Autodesk Inventor part; units mm, degrees
ref_plane "YZ Plane" through (0, 0, 0) normal (1, 0, 0) x (0, 1, 0)
ref_plane "XZ Plane" through (0, 0, 0) normal (0, 1, 0) x (-1, 0, 0)
ref_plane "XY Plane" through (0, 0, 0) normal (0, 0, 1) x (1, 0, 0)
sketch "Esboço1" plane through (0, 0, 0) normal (0, 1, 0) x (-1, 0, 0)
  line L0 (20, 75) -> (-20, 75)
  line L1 (-20, 75) -> (-20, -75)
  line L2 (-20, -75) -> (20, -75)
  line L3 (20, -75) -> (20, 75)
  line L4 (7.1, 63.25) -> (7.1, 18.19) construction
  circle A0 centre (7.1, 16.44) radius 1.75 construction
  circle A1 centre (7.1, 65) radius 1.75 construction
  line L5 (7.1, 65) -> (7.1, 63.25) construction
  line L6 (7.1, 16.44) -> (7.1, 18.19) construction
  circle A2 centre (7.1, 16.44) radius 1.45
  circle A3 centre (7.1, 65) radius 1.45
  line L7 (14.5, 62.22) -> (-14.5, 62.22) construction
  line L8 (-14.5, 62.22) -> (-14.5, 19.22) construction
  line L9 (-14.5, 19.22) -> (14.5, 19.22) construction
  line L10 (14.5, 19.22) -> (14.5, 62.22) construction
  line L11 (11.1, 61) -> (3.1, 61) construction
  line L12 (3.1, 61) -> (3.1, 69) construction
  line L13 (3.1, 69) -> (11.1, 69) construction
  line L14 (11.1, 69) -> (11.1, 61) construction
  line L15 (11.1, 61) -> (3.1, 69) construction
  line L16 (3.1, 61) -> (11.1, 69) construction
  line L17 (3.1, 20.44) -> (11.1, 20.44) construction
  line L18 (11.1, 20.44) -> (11.1, 12.44) construction
  line L19 (11.1, 12.44) -> (3.1, 12.44) construction
  line L20 (3.1, 12.44) -> (3.1, 20.44) construction
  line L21 (3.1, 20.44) -> (11.1, 12.44) construction
  line L22 (11.1, 20.44) -> (3.1, 12.44) construction
  line L23 (7.1, 40.72) -> (7.6918, 40.72) construction
  line L24 (14.5, 40.72) -> (22.5062, 40.72) construction
  line L25 (7.1, -1.12) -> (7.1, -24.28) construction
  circle A4 centre (7.1, -1.12) radius 1.45
  circle A5 centre (7.1, -24.28) radius 1.45
  circle A6 centre (7.1, -41.84) radius 1.45
  circle A7 centre (7.1, -65) radius 1.45
  line L26 (7.1, -41.84) -> (7.1, -65) construction
  line L27 (7.1, 16.44) -> (7.1, -1.12) construction
  line L28 (7.1, -24.28) -> (7.1, -41.84) construction
  line L29 (0, 62.22) -> (0, 19.22) construction
  line L30 (0, 75) -> (0, 85.6082) construction
  point P0 (0, 0)
  dimension "d5" = 3.5
  dimension "d6" = 3.5
  dimension "d0" = 150
  dimension "d1" = 40
  dimension "d2" = 20
  dimension "d3" = 75
  dimension "d4" = 45.06
  dimension "d7" = 2.9
  dimension "d8" = 2.9
  dimension "d9" = 48.56
  dimension "d10" = 29
  dimension "d11" = 8
  dimension "d12" = 8
  dimension "d13" = 8
  dimension "d14" = 8
  dimension "d15" = 3.4
  dimension "d16" = 43
  dimension "d17" = 2.9
  dimension "d18" = 2.9
  dimension "d19" = 23.16
  dimension "d20" = 2.9
  dimension "d21" = 2.9
  dimension "d22" = 23.16
  dimension "d23" = 10
  dimension "d24" = 10
extrude "Extrusão1" add sketch "Esboço1" along normal blind 10 contours L3 L2 L1 L0 | A2 | A3 | A4 | A5 | A6 | A7
sketch "Esboço2" plane through (0, 10, 0) normal (0, 1, 0) x (1, 0, 0)
  circle A0 centre (-7.1, -65) radius 1.45
  circle A1 centre (-7.1, -16.44) radius 1.45
  circle A2 centre (-7.1, 1.12) radius 1.45
  circle A3 centre (-7.1, 24.28) radius 1.45
  circle A4 centre (-7.1, 41.84) radius 1.45
  circle A5 centre (-7.1, 65) radius 1.45
  point P0 (0, 0)
extrude "Extrusão2" cut sketch "Esboço2" against normal blind 8.5
fillet "Arredondamento1" radius 5 4 edges at (20, 5, 75) (-20, 5, 75) (20, 5, -75) (-20, 5, -75)
equation "\"d12\" = d11"
equation "\"d13\" = d12"
equation "\"d14\" = d12"
equation "\"d17\" = d8"
equation "\"d18\" = d17"
equation "\"d20\" = d18"
equation "\"d21\" = d18"
equation "\"d22\" = d19"
equation "\"d24\" = d23"
properties part number "Base barramentos"
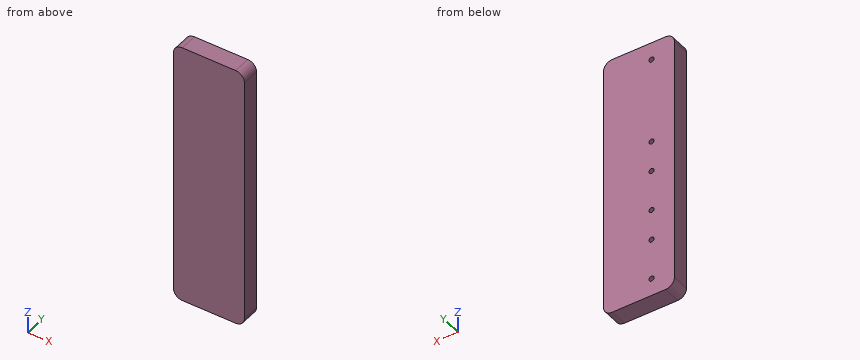
The listing builds one solid part. Answer for the finished solid, in the listing's coordinates (mm). Give positions to 0.01 mm unless a question says otherwise; leave off trailing zeros. Order: outer loops, then holes, each group sorted by start corner. A loop starts at its lowest first (then second) coordinate and runs counter-clockwise, first axis right, second up.
1) Given P1, Ø3, axis at x = -7, z = 16.5, coming from the +Y side; P2, Ø1.4, axis at x = -6.5, z = -24.5, coming from the +Y side, each flat-ended and moving along its own axis, determine where each tip first touches the part or whether it passes through.
Reported:
P1: stops at y = 10
P2: stops at y = 1.5
2) Consider line 1 along X through (y, z) = (6, -41.84); line 2 along Z through (x, y) = (-18, 4.25). Determine where each line is inside the solid, lowest interval first.
Reported:
line 1: x = -20 to -8.55, -5.65 to 20
line 2: z = -74 to 74
3) Find section B-B on x = -7.1. Write down the section's boundary in (y, z), then the cut area to 3 significant figures.
Reported:
outline: (0, -75) - (10, -75) - (10, -66.45) - (1.5, -66.45) - (1.5, -63.55) - (10, -63.55) - (10, -43.29) - (1.5, -43.29) - (1.5, -40.39) - (10, -40.39) - (10, -25.73) - (1.5, -25.73) - (1.5, -22.83) - (10, -22.83) - (10, -2.57) - (1.5, -2.57) - (1.5, 0.33) - (10, 0.33) - (10, 14.99) - (1.5, 14.99) - (1.5, 17.89) - (10, 17.89) - (10, 63.55) - (1.5, 63.55) - (1.5, 66.45) - (10, 66.45) - (10, 75) - (0, 75) - close
area: 1,350 mm2
4) Find section A-A on z = -24.28. Write down the section's boundary in (x, y).
Reported:
outline: (-20, 0) - (20, 0) - (20, 10) - (-5.65, 10) - (-5.65, 1.5) - (-8.55, 1.5) - (-8.55, 10) - (-20, 10) - close
